```python
from build123d import *

# Parameters (mm, degrees)
BOSS_EXTRUDE1_DEPTH = 114.3
CUT_EXTRUDE1_DEPTH  = 6.604
CUT_EXTRUDE3_DEPTH  = 39.354


with BuildPart() as part:
    # Sketch1 → Boss-Extrude1 (new body)
    with BuildSketch(Plane.XY):
        Polygon((7.332348419, 0), (3.666174209, 6.35), (-3.666174209, 6.35), (-7.332348419, 0), (-3.666174209, -6.35), (3.666174209, -6.35), align=None)
    extrude(amount=BOSS_EXTRUDE1_DEPTH)

    # Sketch1_3 → Cut-Extrude1 (cut)
    with BuildSketch(Plane.XY):
        with BuildLine():
            ThreePointArc((-5.499261317, -3.174999996), (-6.35, 5.6e-08), (-5.499261261, 3.175000092))
            Line((-5.499261261, 3.175000092), (-7.332348419, 0))
            Line((-7.332348419, 0), (-5.499261317, -3.174999996))
        make_face()
        with BuildLine():
            ThreePointArc((-5.499261261, 3.175000092), (-3.174999954, 5.499261341), (0, 6.35))
            Line((0, 6.35), (-3.666174209, 6.35))
            Line((-3.666174209, 6.35), (-5.499261261, 3.175000092))
        make_face()
        with BuildLine():
            ThreePointArc((0, 6.35), (3.174999954, 5.499261341), (5.499261261, 3.175000092))
            Line((5.499261261, 3.175000092), (3.666174209, 6.35))
            Line((3.666174209, 6.35), (0, 6.35))
        make_face()
        with BuildLine():
            Line((5.499261261, -3.175000092), (7.332348419, 0))
            Line((7.332348419, 0), (5.499261261, 3.175000092))
            ThreePointArc((5.499261261, 3.175000092), (6.133628983, 1.643500988), (6.35, 0))
            ThreePointArc((6.35, 0), (6.133628983, -1.643500988), (5.499261261, -3.175000092))
        make_face()
        with BuildLine():
            Line((3.666174209, -6.35), (5.499261261, -3.175000092))
            ThreePointArc((5.499261261, -3.175000092), (3.174999954, -5.499261341), (0, -6.35))
            Line((0, -6.35), (3.666174209, -6.35))
        make_face()
        with BuildLine():
            Line((-3.666174209, -6.35), (0, -6.35))
            ThreePointArc((0, -6.35), (-3.175000002, -5.499261313), (-5.499261317, -3.174999996))
            Line((-5.499261317, -3.174999996), (-3.666174209, -6.35))
        make_face()
    extrude(amount=CUT_EXTRUDE1_DEPTH, mode=Mode.SUBTRACT)

    # Sketch3 → Cut-Extrude3 (cut, through all)
    with BuildSketch(Plane(origin=(0, 0, 75.946), x_dir=(-1, 0, 0), z_dir=(0, 0, -1))):
        with BuildLine():
            ThreePointArc((5.499261168, -3.175000253), (3.174999873, -5.499261387), (0, -6.35))
            Line((0, -6.35), (3.666174209, -6.35))
            Line((3.666174209, -6.35), (5.499261168, -3.175000253))
        make_face()
        with BuildLine():
            ThreePointArc((0, -6.35), (-3.17500011, -5.499261251), (-5.499261441, -3.17499978))
            Line((-5.499261441, -3.17499978), (-3.666174209, -6.35))
            Line((-3.666174209, -6.35), (0, -6.35))
        make_face()
        with BuildLine():
            ThreePointArc((-5.499261441, -3.17499978), (-6.35, 0), (-5.499261441, 3.17499978))
            Line((-5.499261441, 3.17499978), (-7.332348419, 0))
            Line((-7.332348419, 0), (-5.499261441, -3.17499978))
        make_face()
        with BuildLine():
            Line((0, 6.35), (-3.666174209, 6.35))
            Line((-3.666174209, 6.35), (-5.499261441, 3.17499978))
            ThreePointArc((-5.499261441, 3.17499978), (-3.17500011, 5.499261251), (0, 6.35))
        make_face()
        with BuildLine():
            Line((3.666174209, 6.35), (0, 6.35))
            ThreePointArc((0, 6.35), (3.175000128, 5.49926124), (5.499261462, 3.174999743))
            Line((5.499261462, 3.174999743), (3.666174209, 6.35))
        make_face()
        with BuildLine():
            Line((7.332348419, 0), (5.499261462, 3.174999743))
            ThreePointArc((5.499261462, 3.174999743), (6.133629035, 1.643500793), (6.35, 0))
            ThreePointArc((6.35, 0), (6.133628959, -1.643501078), (5.499261168, -3.175000253))
            Line((5.499261168, -3.175000253), (7.332348419, 0))
        make_face()
    extrude(amount=-CUT_EXTRUDE3_DEPTH, mode=Mode.SUBTRACT)


solid = part.part
```
Design review of the part built by this model. Coordinates are the model's own, in mm. A direction names the side the tool comes from. Coordinates: 2 decimals unless noted, no trailing zeros. Order: outer loops, then holes, each group sorted by start corner. A loop starts at its lowest first (then second) coordinate and runs counter-clockwise, first axis right, second up. Notation, with made-up numbers: (37.25, 39.25) - (49.25, 39.25) arc R26 cw to (49.25, 74.25) - close; hole circle Ø6 at (4, 75). An arc over 180 degrees is marked (long way). Answer in a Markdown table with one row per item.
(1) Consider section B-B on x = 2.25. State the section outline as (y, z) points, plus the area to 3 significant figures.
Checked values:
| item | result |
|---|---|
| outline | (-6.35, 6.6) - (-5.94, 6.6) - (-5.94, 0) - (5.94, 0) - (5.94, 6.6) - (6.35, 6.6) - (6.35, 75.95) - (5.94, 75.95) - (5.94, 114.3) - (-5.94, 114.3) - (-5.94, 75.95) - (-6.35, 75.95) - close |
| area | 1,410 mm^2 |
(2) Consider section A-A on z = 82. State the section outline as (x, y) points (3 decimals), plus the area to 3 significant figures.
Checked values:
| item | result |
|---|---|
| outline | circle Ø12.7 at (0, 0) |
| area | 127 mm^2 |
(3) Consider section D-D on z = 46. State the section outline as (x, y) points.
Checked values:
| item | result |
|---|---|
| outline | (-7.33, 0) - (-3.67, -6.35) - (3.67, -6.35) - (7.33, 0) - (3.67, 6.35) - (-3.67, 6.35) - close |
(4) Wall thickness on line 1 along Y through (x, z) = (5.5, 57); line 2 along Z through (x, y) = (-6.5, -0.75): over which ranges is each line inside the solid? List them lowest first. Write a range as from..to.
Checked values:
| item | result |
|---|---|
| line 1 | -3.17..3.17 |
| line 2 | 6.6..75.95 |
(5) Consider section C-C on y = 5.25. State the section outline as (x, z) points.
Checked values:
| item | result |
|---|---|
| outline | (-4.3, 6.6) - (-3.57, 6.6) - (-3.57, 0) - (3.57, 0) - (3.57, 6.6) - (4.3, 6.6) - (4.3, 75.95) - (3.57, 75.95) - (3.57, 114.3) - (-3.57, 114.3) - (-3.57, 75.95) - (-4.3, 75.95) - close |
(6) For faces 1 (the flat face through (3, -6, 6.604)), 2 (the flat face through (3, 6, 6.604)), 3 (the flat face through (3, 6, 75.946)), 4 (the flat face through (-3, -6, 6.604)), list the 3-axis set-ups (+Z, -Z, +X, -X, +Y, -Y) from which the entire face can be reached by the end or side of a thin tool; tool diameter is ignored.
Checked values:
| item | result |
|---|---|
| face 1 | -Z, +X, -Y |
| face 2 | -Z, +X, +Y |
| face 3 | +Z, +X, +Y |
| face 4 | -Z, -X, -Y |
(7) Clearance check with flat-ended pins moving along their axes: pin 1 (0.5 mm diameter, centred on x = -6.5, y = 1.5, fed in from +Z); pin 2 (1.6 mm diameter, centred on x = -3.5, y = 5, fed in from -Z); pin 3 (5 mm diameter, centred on x = -4, z = 96.5, fed in from +Y); pin 4 (6 mm diameter, centred on y = -3.5, z = 66.5, fed in from +X). State where each tip first meets the part, or that it passes through.
Checked values:
| item | result |
|---|---|
| pin 1 | z = 75.95 |
| pin 2 | z = 0 |
| pin 3 | y = 6.17 |
| pin 4 | x = 7.04 |
